The listing builds one solid part. Answer for the finished solid, in the listing's coordinates (mm). Face numbers are marked on the shaded views. A direction names the side the tool comes from. Round coordinates to 2 decimals unless told otherwise and drop trailing zeros. Loops run counter-clockwise (first coordinate to the right, second up) from the corner with the lowest first, then second, coordinate; pieces in that order, holes last. Notation, with made-up numbers: M 36,63 L 69,63 A32 cw 69,91 Z; hole C 73.5,-4.75 d1. An arc over 180 degrees is marked long. Put each result on its own line as item: value. Start each with the question number.
(1) Section D-D, the plane y = 3 is taken. Determine the outline of the cut face in (x, z), then the cut area to 3 significant figures.
(2) Section A-A, the plane y = 1.5 is taken. Count the separate pieces of the cut face and the enclosed holes in it, then the cut area to 3 significant figures.
(3) Determine the mould class of the marked faces 4, 5 and 6 for opening direction X: released by +X, released by -X, zero draft, split by the parting line, or undercut.
(4) Which of the six approach directions +Z, -Z, +X, -X, +Y, -Y give full straight-line access (tool end or side, diameter ignored) to the marked faces 1, 2 and 3?
(5) Section C-C, the plane z = 0 is taken. Determine the outline of the cut face in (x, y).
(6) Flat-ended cylindrical pins translate along their axes: P1, Ø3, axis at x = -6.5, y = 2.5, coming from the +Z side; P2, Ø2.5, axis at x = 0, z = 0, coming from the +Y side; P3, Ø1, axis at y = 2.5, z = 1.5, coming from the +X side. Find the tip coordinate at first contact, or state that the pin passes through.
(7) Straight lines are drawn through the part: line 1 (X direction, y = 3.25, z = 0); line 2 (X direction, y = 0.1, z = 0); line 3 (Z direction, x = 3.25, y = -1.5) (3 decimals). For each, find the intervals that lie inside material, in ascending order.
```python
from build123d import *

# Parameters (mm, degrees)
BASES_R               = 8.9
BASE_DEPTH            = 1.2
O_RINGCAPTURES_R      = 6.8
O_RINGCAPTURE_DEPTH   = 3.7
SEALINGFACES_R        = 4.5
SEALINGFACE_DEPTH     = 0.4
SLOTCUTS_W            = 9
SLOTCUTS_H            = 1.5
SLOTCUT_DEPTH         = 0.4
BOTTOMBASES_R         = 7.8
BOTTOMBASE_DEPTH      = 0.8
TOPBORES_R            = 1.7
TOPBORE_DEPTH         = 1.4
BOTTOMBORES_R         = 5.5
BOTTOMBORE_DEPTH      = 4.4
CENTRALCYLINDERS_R    = 2.5
CENTRALCYLINDER_DEPTH = 2.6
CYLINDERBORES_R       = 1.5
CYLINDERBORE_DEPTH    = 0.6
RIB_REACH             = 15.333
RIBCP_COUNT           = 8
RIBCUTS_W             = 1.25
RIBCUTS_H             = 3.3
RIBCUT_DEPTH          = 0.2
RIBCUTCP_COUNT        = 4


with BuildPart() as part:
    # BaseS → Base (new body)
    with BuildSketch(Plane(origin=(0, 0, 0), x_dir=(1, 0, 0), z_dir=(0, 1, 0))):
        with Locations(Location((0, 0, 0), (0, 0, 270))):
            Circle(BASES_R)
    extrude(amount=-BASE_DEPTH)

    # O-RingCaptureS → O-RingCapture (add)
    with BuildSketch(Plane(origin=(0, 0, 0), x_dir=(1, 0, 0), z_dir=(0, 1, 0))):
        with Locations(Location((0, 0, 0), (0, 0, 270))):
            Circle(O_RINGCAPTURES_R)
    extrude(amount=O_RINGCAPTURE_DEPTH)

    # SealingFaceS → SealingFace (add)
    with BuildSketch(Plane(origin=(0, 3.7, 0), x_dir=(1, 0, 0), z_dir=(0, 1, 0))):
        with Locations(Location((0, 0, 0), (0, 0, 270))):
            Circle(SEALINGFACES_R)
    extrude(amount=SEALINGFACE_DEPTH)

    # SlotCutS → SlotCut (cut)
    with BuildSketch(Plane(origin=(0, 4.1, 0), x_dir=(1, 0, 0), z_dir=(0, 1, 0))):
        Rectangle(SLOTCUTS_W, SLOTCUTS_H)
    extrude(amount=-SLOTCUT_DEPTH, mode=Mode.SUBTRACT)

    # BottomBaseS → BottomBase (add)
    with BuildSketch(Plane.XZ.offset(1.2)):
        with Locations(Location((0, 0, 0), (0, 0, 270))):
            Circle(BOTTOMBASES_R)
    extrude(amount=BOTTOMBASE_DEPTH)

    # TopBoreS → TopBore (cut)
    with BuildSketch(Plane(origin=(0, 4.1, 0), x_dir=(1, 0, 0), z_dir=(0, 1, 0))):
        with Locations(Location((0, 0, 0), (0, 0, 270))):
            Circle(TOPBORES_R)
    extrude(amount=-TOPBORE_DEPTH, mode=Mode.SUBTRACT)

    # BottomBoreS → BottomBore (cut)
    with BuildSketch(Plane.XZ.offset(2)):
        with Locations(Location((0, 0, 0), (0, 0, 270))):
            Circle(BOTTOMBORES_R)
    extrude(amount=-BOTTOMBORE_DEPTH, mode=Mode.SUBTRACT)

    # CentralCylinderS → CentralCylinder (add)
    with BuildSketch(Plane(origin=(0, 2.4, 0), x_dir=(-1, 0, 0), z_dir=(0, -1, 0))):
        with Locations(Location((0, 0, 0), (0, 0, 90))):
            Circle(CENTRALCYLINDERS_R)
    extrude(amount=CENTRALCYLINDER_DEPTH)

    # CylinderBoreS → CylinderBore (cut)
    with BuildSketch(Plane(origin=(0, -0.2, 0), x_dir=(-1, 0, 0), z_dir=(0, -1, 0))):
        with Locations(Location((0, 0, 0), (0, 0, 90))):
            Circle(CYLINDERBORES_R)
    extrude(amount=-CYLINDERBORE_DEPTH, mode=Mode.SUBTRACT)

    # Rib: up to this face of the body (flat: up to its plane)
    rib_end = Plane(part.part.faces().sort_by_distance((0, -2, 7.579382684))[0])
    # RibS → Rib (add, up to the picked face)
    with BuildSketch(Plane(origin=(0, 2.4, 0), x_dir=(-1, 0, 0), z_dir=(0, -1, 0)), mode=Mode.PRIVATE) as rib_sk1:
        with BuildLine():
            Line((0.625, -5.464373249), (0.625, -2.420614591))
            ThreePointArc((0.625, -2.420614591), (0, -2.5), (-0.625, -2.420614591))
            Line((-0.625, -2.420614591), (-0.625, -5.464373249))
            ThreePointArc((-0.625, -5.464373249), (0, -5.5), (0.625, -5.464373249))
        make_face()
    rib_tool1 = split(extrude(rib_sk1.sketch, amount=RIB_REACH, mode=Mode.PRIVATE), bisect_by=rib_end, keep=Keep.BOTH, mode=Mode.PRIVATE)
    rib = rib_tool1.solids().sort_by(Axis((0, 2.4, 3.98085), (0, -1, 0)))[0]
    add(rib)

    # RibCP: Rib ×8 about axis
    ribcp_axis = Axis((0, 0, 0), (0, 1, 0))
    for i in range(1, RIBCP_COUNT):
        add(rib.rotate(ribcp_axis, i * 360 / RIBCP_COUNT))

    # RibCutS → RibCut (cut)
    with BuildSketch(Plane.XZ.offset(2)):
        with Locations((0, 6.15)):
            Rectangle(RIBCUTS_W, RIBCUTS_H)
    ribcut = extrude(amount=-RIBCUT_DEPTH, mode=Mode.SUBTRACT)

    # RibCutCP: RibCut ×4 about axis
    ribcutcp_axis = Axis((0, 0, 0), (0, 1, 0))
    for i in range(1, RIBCUTCP_COUNT):
        add(ribcut.rotate(ribcutcp_axis, i * 360 / RIBCUTCP_COUNT), mode=Mode.SUBTRACT)


solid = part.part
```
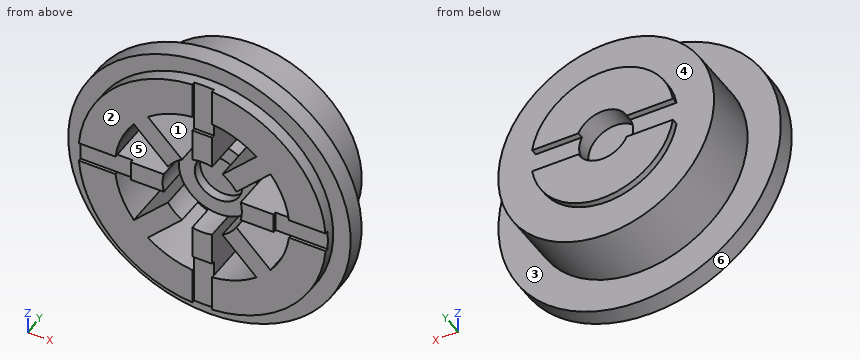
Recorded:
1. outline: C 0,0 d13.6; hole C 0,0 d3.4
1. area: 136 mm²
2. separate pieces: 1
2. enclosed holes: 8
2. area: 100 mm²
3. face 4: zero draft
3. face 5: undercut
3. face 6: split by the parting line
4. face 1: -Y
4. face 2: +Z, -Z, +X, -X, -Y
4. face 3: +Y
5. outline: M -8.9,-1.2 L -7.8,-1.2 L -7.8,-1.8 L -4.5,-1.8 L -4.5,-2 L -2.5,-2 L -2.5,-0.2 L -1.5,-0.2 L -1.5,0.4 L 1.5,0.4 L 1.5,-0.2 L 2.5,-0.2 L 2.5,-2 L 4.5,-2 L 4.5,-1.8 L 7.8,-1.8 L 7.8,-1.2 L 8.9,-1.2 L 8.9,0 L 6.8,0 L 6.8,3.7 L 1.7,3.7 L 1.7,2.7 L -1.7,2.7 L -1.7,3.7 L -6.8,3.7 L -6.8,0 L -8.9,0 Z
6. P1: stops at z = 4.61
6. P2: stops at y = 2.7
6. P3: stops at x = 6.73
7. line 1: x = -6.8 to -1.7, 1.7 to 6.8
7. line 2: x = -6.8 to -1.5, 1.5 to 6.8
7. line 3: z = -7.091 to -4.437, -4.134 to -2.366, -0.625 to 0.625, 2.366 to 4.134, 4.437 to 7.091
